```python
from build123d import *

# Parameters (mm, degrees)
SKETCH2_W                                     = 304.8
SKETCH2_H                                     = 254
BOSS_EXTRUDE1_DEPTH                           = 6.35
SKETCH3_R                                     = 3.96875
CUT_EXTRUDE1_DEPTH                            = 199.481945023
CSK_FOR_1_4_FLAT_HEAD_MACHINE_SCREW1_AT_COUNT = 2
CSK_FOR_1_4_FLAT_HEAD_MACHINE_SCREW1_AT_PITCH = 228.6
CSK_FOR_1_4_FLAT_HEAD_MACHINE_SCREW1_2_COUNT  = 2
CSK_FOR_1_4_FLAT_HEAD_MACHINE_SCREW1_2_PITCH  = 323.289220358
CSK_FOR_1_4_FLAT_HEAD_MACHINE_SCREW1_3_COUNT  = 2
CSK_FOR_1_4_FLAT_HEAD_MACHINE_SCREW1_3_PITCH  = 228.6
CSK_FOR_1_4_FLAT_HEAD_MACHINE_SCREW1_4_COUNT  = 2
CSK_FOR_1_4_FLAT_HEAD_MACHINE_SCREW1_4_PITCH  = 209.55
CSK_FOR_1_4_FLAT_HEAD_MACHINE_SCREW1_5_COUNT  = 2
CSK_FOR_1_4_FLAT_HEAD_MACHINE_SCREW1_5_PITCH  = 238.695815841
CSK_FOR_1_4_FLAT_HEAD_MACHINE_SCREW1_6_COUNT  = 2
CSK_FOR_1_4_FLAT_HEAD_MACHINE_SCREW1_6_PITCH  = 310.111532356
CSK_FOR_1_4_FLAT_HEAD_MACHINE_SCREW1_7_COUNT  = 2
CSK_FOR_1_4_FLAT_HEAD_MACHINE_SCREW1_7_PITCH  = 25.4
CSK_FOR_1_4_FLAT_HEAD_MACHINE_SCREW1_8_COUNT  = 2
CSK_FOR_1_4_FLAT_HEAD_MACHINE_SCREW1_8_PITCH  = 203.2
F_10_32_TAPPED_HOLE1_D                        = 4.0386
F_10_32_TAPPED_HOLE1_CSINK_D                  = 6.096
F_10_32_TAPPED_HOLE1_CSINK_ANGLE              = 90


with BuildPart() as part:
    # Sketch2 → Boss-Extrude1 (new body)
    with BuildSketch(Plane(origin=(0, 0, 0), x_dir=(1, 0, 0), z_dir=(0, 1, 0))):
        Rectangle(SKETCH2_W, SKETCH2_H)
    extrude(amount=BOSS_EXTRUDE1_DEPTH)

    # Sketch3 → Cut-Extrude1 (cut, through all)
    with BuildSketch(Plane(origin=(0, 6.35, 0), x_dir=(1, 0, 0), z_dir=(0, 1, 0))):
        with Locations(Location((139.7, 114.3, 0), (0, 0, 270))):
            Circle(SKETCH3_R)
        with Locations(Location((139.7, -114.3, 0), (0, 0, 90))):
            Circle(SKETCH3_R)
        with Locations(Location((-139.7, 114.3, 0), (0, 0, 90))):
            Circle(SKETCH3_R)
        with Locations(Location((-139.7, -114.3, 0), (0, 0, 270))):
            Circle(SKETCH3_R)
    extrude(amount=-CUT_EXTRUDE1_DEPTH, mode=Mode.SUBTRACT)

    # Sketch5 → CSK for 1/4 Flat Head Machine Screw1 (revolve, cut)
    with BuildSketch(Plane(origin=(-114.3, 0, -114.3), x_dir=(0, 0, -1), z_dir=(1, 0, 0))):
        Polygon((0, 0), (0, 6.35), (3.3782, 6.35), (3.3782, 3.520932584), (6.4389, 0), align=None)
    csk_for_1_4_flat_head_machine_screw1 = revolve(axis=Axis((-114.3, -6.35, -114.3), (0, 1, 0)), mode=Mode.SUBTRACT)

    # CSK for 1/4 Flat Head Machine Screw1 at: CSK for 1/4 Flat Head Machine Screw1 ×2
    with Locations(*[(0, 0, i * CSK_FOR_1_4_FLAT_HEAD_MACHINE_SCREW1_AT_PITCH) for i in range(1, CSK_FOR_1_4_FLAT_HEAD_MACHINE_SCREW1_AT_COUNT)]):
        add(csk_for_1_4_flat_head_machine_screw1, mode=Mode.SUBTRACT)

    # CSK for 1_4 Flat Head Machine Screw1 2: CSK for 1/4 Flat Head Machine Screw1 ×2
    with Locations(*[Vector(0.7071067811865474, 0, 0.7071067811865477) * (i * CSK_FOR_1_4_FLAT_HEAD_MACHINE_SCREW1_2_PITCH) for i in range(1, CSK_FOR_1_4_FLAT_HEAD_MACHINE_SCREW1_2_COUNT)]):
        add(csk_for_1_4_flat_head_machine_screw1, mode=Mode.SUBTRACT)

    # CSK for 1_4 Flat Head Machine Screw1 3: CSK for 1/4 Flat Head Machine Screw1 ×2
    with Locations(*[(i * CSK_FOR_1_4_FLAT_HEAD_MACHINE_SCREW1_3_PITCH, 0, 0) for i in range(1, CSK_FOR_1_4_FLAT_HEAD_MACHINE_SCREW1_3_COUNT)]):
        add(csk_for_1_4_flat_head_machine_screw1, mode=Mode.SUBTRACT)

    # CSK for 1_4 Flat Head Machine Screw1 4: CSK for 1/4 Flat Head Machine Screw1 ×2
    with Locations(*[(i * CSK_FOR_1_4_FLAT_HEAD_MACHINE_SCREW1_4_PITCH, 0, 0) for i in range(1, CSK_FOR_1_4_FLAT_HEAD_MACHINE_SCREW1_4_COUNT)]):
        add(csk_for_1_4_flat_head_machine_screw1, mode=Mode.SUBTRACT)

    # CSK for 1_4 Flat Head Machine Screw1 5: CSK for 1/4 Flat Head Machine Screw1 ×2
    with Locations(*[Vector(0.8778955729143844, 0, 0.47885213068057336) * (i * CSK_FOR_1_4_FLAT_HEAD_MACHINE_SCREW1_5_PITCH) for i in range(1, CSK_FOR_1_4_FLAT_HEAD_MACHINE_SCREW1_5_COUNT)]):
        add(csk_for_1_4_flat_head_machine_screw1, mode=Mode.SUBTRACT)

    # CSK for 1_4 Flat Head Machine Screw1 6: CSK for 1/4 Flat Head Machine Screw1 ×2
    with Locations(*[Vector(0.6757246285173463, 0, 0.7371541402007415) * (i * CSK_FOR_1_4_FLAT_HEAD_MACHINE_SCREW1_6_PITCH) for i in range(1, CSK_FOR_1_4_FLAT_HEAD_MACHINE_SCREW1_6_COUNT)]):
        add(csk_for_1_4_flat_head_machine_screw1, mode=Mode.SUBTRACT)

    # CSK for 1_4 Flat Head Machine Screw1 7: CSK for 1/4 Flat Head Machine Screw1 ×2
    with Locations(*[(0, 0, i * CSK_FOR_1_4_FLAT_HEAD_MACHINE_SCREW1_7_PITCH) for i in range(1, CSK_FOR_1_4_FLAT_HEAD_MACHINE_SCREW1_7_COUNT)]):
        add(csk_for_1_4_flat_head_machine_screw1, mode=Mode.SUBTRACT)

    # CSK for 1_4 Flat Head Machine Screw1 8: CSK for 1/4 Flat Head Machine Screw1 ×2
    with Locations(*[(0, 0, i * CSK_FOR_1_4_FLAT_HEAD_MACHINE_SCREW1_8_PITCH) for i in range(1, CSK_FOR_1_4_FLAT_HEAD_MACHINE_SCREW1_8_COUNT)]):
        add(csk_for_1_4_flat_head_machine_screw1, mode=Mode.SUBTRACT)

    # #10-32 Tapped Hole1 (through all)
    with Locations(Plane(origin=(0, 6.35, 0), x_dir=(1, 0, 0), z_dir=(0, 1, 0))):
        with Locations((114.3, -88.9), (114.3, -63.5), (114.3, 63.5), (114.3, 88.9), (-114.3, 63.5), (-114.3, 38.1), (-114.3, -63.5), (-114.3, -38.1)):
            CounterSinkHole(F_10_32_TAPPED_HOLE1_D / 2, F_10_32_TAPPED_HOLE1_CSINK_D / 2, counter_sink_angle=F_10_32_TAPPED_HOLE1_CSINK_ANGLE)


solid = part.part
```
Design review of the part built by this model. Coordinates are the model's own, in mm. Coordinates: 2 decimals unless noted, no trailing zeros. Order: outer loops, then holes, each group sorted by start corner. A loop starts at its lowest first (then second) coordinate and runs counter-clockwise, first axis right, second up. Notation, with made-up numbers: (45.25, 14.25) -> (54.25, 14.25) arc R27 cw to (54.25, 51.25) -> close; hole circle Ø3 at (80.25, 29). An arc over 180 degrees is marked (long way). One line per item, written item: value. Start each with the question number.
Q1. Take a section at A-A, the plane x = 139.7. State the section outline as (y, z) points.
Q2. For probe 1 along X at (y, z) = (5.5, 114.3); probe 2 along X at (y, z) = (4.75, 0); probe 3 along X at (y, z) = (1.5, 88), list the stretches that pass through material, from the lowest coordinate up.
Q3. Insertion check: pin 1 Ø4.5 at (x, z) = (114.3, 63.5) entering from +Y; pin 2 Ø5.5 at (x, z) = (-114.3, -63.5) entering from +Y; pin 3 Ø8 at (x, z) = (-114.3, -88.9) entering from -Y. Each pin has a flat end and moves straight along its axis. Give the tip position at first contact, or say it passes through.
Q4. Take a section at B-B, the plane z = 114.3. Give the number of separate pieces and of enclosed holes in the cut face, then the cut area to 3 significant figures.
Q5. Mouldability with a two-part tool opening along Z and no side actions: class faces 1 (the flat face through (-2, 3, 127)), 2 (the flat face through (152.4, 3, 2)), 3 (the conical face through (92.24, 3.3, 112.38)) as pulls with the +Z half, pulls with the -Z half, needs draft (parallel to the pull), parting line crosses it, or undercut.
Values follow:
1. outline: (0, -127) -> (6.35, -127) -> (6.35, -118.27) -> (0, -118.27) -> close; (0, -110.33) -> (6.35, -110.33) -> (6.35, 110.33) -> (0, 110.33) -> close; (0, 118.27) -> (6.35, 118.27) -> (6.35, 127) -> (0, 127) -> close
2. probe 1: x = -152.4 to -143.67, -135.73 to -117.68, -110.92 to 91.87, 98.63 to 110.92, 117.68 to 135.73, 143.67 to 152.4
2. probe 2: x = -152.4 to 91.87, 98.63 to 152.4
2. probe 3: x = -152.4 to -119.36, -109.24 to 112.49, 116.11 to 152.4
3. pin 1: stops at y = 5.55
3. pin 2: stops at y = 6.05
3. pin 3: stops at y = 2.81
4. separate pieces: 6
4. enclosed holes: 0
4. area: 1,670 mm2
5. face 1: pulls with the +Z half
5. face 2: needs draft
5. face 3: undercut
